Input: part model. Units: mm. Frame: model coordinates. A direction names the side the tool comes from. Round coordinates to 2 decimals unless told otherwise and drop trailing zeros. Loops run counter-clockwise (first coordinate to the right, second up) from the corner with the lowest first, then second, coordinate; pieces in that order, holes last. Notation, with made-up numbers: (72, 17) -> (121, 17) arc R20 cw to (121, 27) -> close; hole circle Ø11 at (25.25, 57.25). An arc over 180 degrees is marked (long way). Answer as a JSON object with one key per item and string values. Group by question number.
Item 1: Set-up query: faces 5 (the flat face through (21.684, 15, 6)), 6 (the flat face through (-27, 14, 2.75)), 7 (the cylindrical face through (24.2, 25.5, 5.7)). Return all of +Z, -Z, +X, -X, +Y, -Y with unobstructed straight access to the full face (end or side cutting, diameter ignored); none if empty.
Item 2: Section query A-A on y = 24. Return loops of the section in (x, z), and give its area (3 significant figures).
Item 3: Material intervals for line 1 (Y direction, x = 24.5, z = 5.75); line 2 (X direction, y = 23.5, z = 10.25); line 3 (Z direction, x = 24, y = 24), sorted ascending. Write a range as [from, to].
Item 4: Section query B-B on y = 12. Return loops of the section in (x, z).
Item 5: Pin query (flat end, axial travel): pin 1 (2.5 mm diameter, centred on y = 12, z = 5.75, fed in from -X); pin 2 (3.5 mm diameter, centred on y = 24, z = 5.75, fed in from -X). Return the tip coordinate at first contact, or that it passes through.
Item 6: Draft query along Z for faces 1 (the flat face through (-0.9, -0.4, 0)), 2 (the flat face through (-0.9, -0.4, 11.5)), 3 (the flat face through (-28.316, 13, 2)), 4 (the cylindrical face through (-24.584, 12.737, 6.426)). Return one class per face: released by +Z, released by -Z, zero draft, split by the parting line, or undercut.
Item 7: Section query C-C on y = 3. Return loops of the section in (x, z).
Item 8: Section query D-D on x = -11.5. Return loops of the section in (y, z), and give its area (3 significant figures).
from build123d import *

# Parameters (mm, degrees)
F1_DEPTH = 11.5
F3_DEPTH = 25
F4_DEPTH = 2.5
F6_DEPTH = 25


with BuildPart() as f1:
    # F0 (on Top) → F1 (new body)
    with BuildSketch(Plane.XY):
        Polygon((21.6838430613, 0), (-23.3161569387, 0), (-23.3161569387, 30), (-28.3161569387, 30), (-28.3161569387, -5), (26.6838430613, -5), (26.6838430613, 30), (21.6838430613, 30), align=None)
    extrude(amount=F1_DEPTH)

    # F2 (on face) → F3 (cut)
    with BuildSketch(Plane(origin=(-28.3161569387, 0, 0), x_dir=(0, -1, 0), z_dir=(-1, 0, 0))):
        with BuildLine():
            ThreePointArc((-21.75, 2.75), (-20.6458980338, 4.0729490169), (-20.25, 5.75))
            Line((-20.25, 5.75), (-24.0342449397, 5.75))
            Line((-24.0342449397, 5.75), (-24.0342449397, 2.75))
            Line((-24.0342449397, 2.75), (-21.75, 2.75))
        make_face()
        with BuildLine():
            Line((-24.0342449397, 5.75), (-20.25, 5.75))
            ThreePointArc((-20.25, 5.75), (-20.6458980338, 7.4270509831), (-21.75, 8.75))
            Line((-21.75, 8.75), (-24.0342449397, 8.75))
            Line((-24.0342449397, 8.75), (-24.0342449397, 5.75))
        make_face()
        with BuildLine():
            Line((-24.0342449397, 8.75), (-21.75, 8.75))
            ThreePointArc((-21.75, 8.75), (-25.6770509831, 9.1041019662), (-27.75, 5.75))
            Line((-27.75, 5.75), (-24.0342449397, 5.75))
            Line((-24.0342449397, 5.75), (-24.0342449397, 8.75))
        make_face()
        with BuildLine():
            ThreePointArc((-27.75, 5.75), (-25.6770509831, 2.3958980338), (-21.75, 2.75))
            Line((-21.75, 2.75), (-24.0342449397, 2.75))
            Line((-24.0342449397, 2.75), (-24.0342449397, 5.75))
            Line((-24.0342449397, 5.75), (-27.75, 5.75))
        make_face()
        with BuildLine():
            ThreePointArc((-13, 5.75), (-12, 4.75), (-11, 5.75))
            Line((-11, 5.75), (-13, 5.75))
        make_face()
        with BuildLine():
            Line((-13, 5.75), (-11, 5.75))
            ThreePointArc((-11, 5.75), (-12, 6.75), (-13, 5.75))
        make_face()
    extrude(amount=-F3_DEPTH, mode=Mode.SUBTRACT)

    # F2 (on face) → F4 (cut)
    with BuildSketch(Plane(origin=(-28.3161569387, 0, 0), x_dir=(0, -1, 0), z_dir=(-1, 0, 0))):
        with BuildLine():
            Line((-6, 5.75), (-11, 5.75))
            ThreePointArc((-11, 5.75), (-12, 4.75), (-13, 5.75))
            Line((-13, 5.75), (-20.25, 5.75))
            ThreePointArc((-20.25, 5.75), (-20.6458980338, 4.0729490169), (-21.75, 2.75))
            Line((-21.75, 2.75), (-6, 2.75))
            Line((-6, 2.75), (-6, 5.75))
        make_face()
        with BuildLine():
            ThreePointArc((-13, 5.75), (-12, 6.75), (-11, 5.75))
            Line((-11, 5.75), (-6, 5.75))
            Line((-6, 5.75), (-6, 8.75))
            Line((-6, 8.75), (-21.75, 8.75))
            ThreePointArc((-21.75, 8.75), (-20.6458980338, 7.4270509831), (-20.25, 5.75))
            Line((-20.25, 5.75), (-13, 5.75))
        make_face()
    extrude(amount=-F4_DEPTH, mode=Mode.SUBTRACT)

    # F5 (on face) → F6 (cut)
    with BuildSketch(Plane.YZ.offset(26.6838430613)):
        with BuildLine():
            Line((22.5, 5.75), (25.5, 5.75))
            ThreePointArc((25.5, 5.75), (24, 7.25), (22.5, 5.75))
        make_face()
        with BuildLine():
            ThreePointArc((22.5, 5.75), (24, 4.25), (25.5, 5.75))
            Line((25.5, 5.75), (22.5, 5.75))
        make_face()
    extrude(amount=-F6_DEPTH, mode=Mode.SUBTRACT)


solid = f1.part
Solved:
{
 "1": {"face 5": "+Z, -Z, +Y", "face 6": "-X", "face 7": "+X, -X"},
 "2": {"outline": "(-28.32, 0) -> (-23.32, 0) -> (-23.32, 2) -> (-28.32, 2) -> close; (-28.32, 9.5) -> (-23.32, 9.5) -> (-23.32, 11.5) -> (-28.32, 11.5) -> close; (21.68, 0) -> (26.68, 0) -> (26.68, 4.25) -> (21.68, 4.25) -> close; (21.68, 7.25) -> (26.68, 7.25) -> (26.68, 11.5) -> (21.68, 11.5) -> close", "area": "62.5 mm²"},
 "3": {"line 1": "[-5, 22.5], [25.5, 30]", "line 2": "[-28.32, -23.32], [21.68, 26.68]", "line 3": "[0, 4.25], [7.25, 11.5]"},
 "4": {"outline": "(-28.32, 0) -> (-23.32, 0) -> (-23.32, 4.75) -> (-25.82, 4.75) -> (-25.82, 2.75) -> (-28.32, 2.75) -> close; (-28.32, 8.75) -> (-25.82, 8.75) -> (-25.82, 6.75) -> (-23.32, 6.75) -> (-23.32, 11.5) -> (-28.32, 11.5) -> close; (21.68, 0) -> (26.68, 0) -> (26.68, 11.5) -> (21.68, 11.5) -> close"},
 "5": {"pin 1": "x = -25.82", "pin 2": "x = 21.68"},
 "6": {"face 1": "released by -Z", "face 2": "released by +Z", "face 3": "zero draft", "face 4": "undercut"},
 "7": {"outline": "(-28.32, 0) -> (-23.32, 0) -> (-23.32, 11.5) -> (-28.32, 11.5) -> close; (21.68, 0) -> (26.68, 0) -> (26.68, 11.5) -> (21.68, 11.5) -> close"},
 "8": {"outline": "(-5, 0) -> (0, 0) -> (0, 11.5) -> (-5, 11.5) -> close", "area": "57.5 mm²"}
}
